Autodesk Inventor part; units mm, degrees
ref_plane "Work Plane1" through (0, 70, 0) normal (0, 1, 0) x (1, 0, 0)
ref_plane "YZ Plane" through (0, 0, 0) normal (1, 0, 0) x (0, 1, 0)
ref_plane "XZ Plane" through (0, 0, 0) normal (0, 1, 0) x (-1, 0, 0)
sketch "Sketch1" plane through (0, 0, 0) normal (0, 1, 0) x (-1, 0, 0)
  arc A0 (0, 30.16) -> (-3.6283, 29.941) centre (0, 0) ccw construction
  arc A1 (-26.9832, 26.9832) -> (-36.0277, -12.5774) centre (0, 0) ccw construction
  line L0 (38.16, 38.16) -> (0, 38.16) construction
  line L1 (-38.16, 38.16) -> (-38.16, -38.16)
  line L2 (-38.16, -38.16) -> (-4.1245, -38.16)
  line L3 (38.16, -38.16) -> (38.16, 38.16) construction
  line L4 (38.16, 38.16) -> (-21.3263, -21.3263) construction
  line L5 (-38.16, 38.16) -> (-21.3263, 21.3263) construction
  line L6 (0, 38.16) -> (-4.1245, 38.16) construction
  line L7 (0, -38.16) -> (38.16, -38.16) construction
  arc A2 (0, 38.16) -> (-26.9832, 26.9832) centre (0, 0) ccw construction
  arc A3 (-36.9415, -9.566) -> (-26.9832, -26.9832) centre (0, 0) ccw construction
  arc A4 (-26.9832, -26.9832) -> (0, -38.16) centre (0, 0) ccw construction
  arc A5 (0, -38.16) -> (0, 38.16) centre (0, 0) ccw construction
  line L8 (-21.3263, 21.3263) -> (38.16, -38.16) construction
  line L9 (-21.3263, -21.3263) -> (-38.16, -38.16) construction
  line L10 (0, 38.16) -> (0, 30.16) construction
  line L11 (0, -30.16) -> (0, -38.16) construction
  arc A6 (21.3263, 21.3263) -> (0, 30.16) centre (0, 0) ccw construction
  arc A7 (0, -30.16) -> (21.3263, 21.3263) centre (0, 0) ccw construction
  arc A8 (-6.0651, -37.6749) -> (-3.6283, -29.941) centre (-4.1245, -34.0355) ccw
  arc A9 (-3.6283, 29.941) -> (-6.0651, 37.6749) centre (-4.1245, 34.0355) ccw
  line L12 (-4.1245, -38.16) -> (0, -38.16) construction
  arc A10 (-3.6283, -29.941) -> (0, -30.16) centre (0, 0) ccw construction
  arc A11 (-3.6283, 29.941) -> (-3.6283, -29.941) centre (0, 0) ccw
  line L13 (-4.1245, 38.16) -> (-38.16, 38.16)
  arc A12 (-3.6283, -29.941) -> (-6.0651, -37.6749) centre (-4.1245, -34.0355) ccw construction
  arc A13 (-6.0651, 37.6749) -> (-3.6283, 29.941) centre (-4.1245, 34.0355) ccw construction
  dimension "d0" = 60.32
  dimension "d1" = 8
extrude "Extrusion1" add sketch "Sketch1" along normal blind 140
sketch "Sketch2" plane through (38.16, 0, 38.16) normal (1, 0, 0) x (0, 0, -1)
  line L0 (8.219, 140) -> (0, 140)
  line L1 (0, 140) -> (76.32, 0) construction
  line L2 (76.32, 140) -> (0, 0) construction
  circle A0 centre (38.16, 70) radius 25.4
  dimension "d15" = 50.8
extrude "Extrusion2" cut sketch "Sketch2" against normal up to next
ref_plane "Work Plane1" through (0, 70, 0) normal (0, 1, 0) x (1, 0, 0)
sketch "Sketch3" plane through (0, 70, 0) normal (0, 1, 0) x (1, 0, 0)
  line L0 (38.16, 38.16) -> (4.1245, 38.16)
  line L1 (38.16, 25.4) -> (16.2624, 25.4)
  line L2 (38.16, -38.16) -> (38.16, 38.16)
  line L3 (38.16, -25.4) -> (16.2624, -25.4)
  line L4 (4.1245, -38.16) -> (38.16, -38.16)
  line L5 (16.2624, 25.4) -> (38.16, 38.16) construction
  line L6 (38.16, 25.4) -> (16.2624, 38.16) construction
  line L7 (16.2624, -25.4) -> (38.16, -38.16) construction
  line L8 (38.16, -25.4) -> (16.2624, -38.16) construction
  circle A0 centre (27.2112, 31.78) radius 2.5
  circle A1 centre (27.2112, -31.78) radius 2.5
  dimension "d16" = 5
  dimension "d17" = 5
extrude "Extrusion3" cut sketch "Sketch3" along normal through all both and the other way through all
sketch "Sketch5" plane through (38.16, 0, 38.16) normal (1, 0, 0) x (0, 0, -1)
  circle A0 centre (38.16, 70) radius 25.4
  line L0 (0, 140) -> (76.32, 140)
  line L1 (0, 0) -> (76.32, 0)
  line L2 (38.16, 95.4) -> (38.16, 140) construction
  line L3 (38.16, 44.6) -> (38.16, 0) construction
  circle A1 centre (38.16, 112.125) radius 2.55
  circle A2 centre (38.16, 27.875) radius 2.55
  line L4 (38.16, 22.3) -> (38.16, 44.6) construction
  line L5 (38.16, 117.7) -> (38.16, 95.4) construction
  line L6 (38.16, 22.3) -> (38.16, 33.45)
  line L7 (38.16, 117.7) -> (38.16, 106.55)
  dimension "d18" = 5.1
  dimension "d19" = 5.1
extrude "Extrusion4" cut sketch "Sketch5" against normal up to next contours A1 L7 | L7 A1 | A2 L6 | L6 A2
ref_plane "Work Plane2" through (4.1245, 0, 0) normal (0, 0, 1) x (1, 0, 0)
sketch "Sketch7" plane through (38.16, 0, 38.16) normal (1, 0, 0) x (0, 0, -1)
  line L0 (0, 0) -> (0, 140) construction
  line L1 (0, 140) -> (0, 0) construction
  line L2 (0, 89) -> (0, 51)
  circle A0 centre (-4, 93) radius 4 construction
  circle A1 centre (-4, 93) radius 2.75
  circle A2 centre (-4, 85) radius 4 construction
  circle A3 centre (-4, 85) radius 2.75
  arc A4 (-12.9282, 85.5359) -> (-12.9282, 92.4641) centre (-10.9282, 89) ccw construction
  circle A5 centre (-10.9282, 89) radius 2.75
  line L3 (0, 70) -> (-10, 70) construction
  line L4 (0, 89) -> (-10, 89) construction
  line L5 (0, 78.0718) -> (-12.9282, 85.5359)
  line L6 (-12.9282, 92.4641) -> (0, 99.9282)
  arc A6 (-12.9282, 92.4641) -> (-12.9282, 85.5359) centre (-10.9282, 89) ccw
  circle A7 centre (-4, 47) radius 4 construction
  circle A8 centre (-4, 47) radius 2.75
  circle A9 centre (-4, 55) radius 4 construction
  circle A10 centre (-4, 55) radius 2.75
  arc A11 (-12.9282, 47.5359) -> (-12.9282, 54.4641) centre (-10.9282, 51) ccw construction
  circle A12 centre (-10.9282, 51) radius 2.75
  line L7 (0, 51) -> (-10, 51) construction
  line L8 (0, 61.9282) -> (-12.9282, 54.4641)
  line L9 (-12.9282, 47.5359) -> (0, 40.0718)
  arc A13 (-12.9282, 54.4641) -> (-12.9282, 47.5359) centre (-10.9282, 51) ccw
  line L10 (0, 89) -> (0, 99.9282)
  line L11 (0, 51) -> (0, 40.0718)
  point P0 (38.16, 0)
  dimension "d26" = 38
  dimension "d27" = 8
  dimension "d28" = 5.5
  dimension "d29" = 8
  dimension "d30" = 5.5
  dimension "d31" = 8
  dimension "d32" = 5.5
  dimension "d33" = 10
  dimension "d34" = 10
extrude "Extrusion6" add sketch "Sketch7" against normal blind 125.446
properties part number "Tubo Exterior" material "ABS Plastic"
Read the model definition and answer for the solid it produces. Units are mm, in the model's axes. A direction names the side the tool comes from. Coordinates: 2 decimals unless noted, no trailing zeros. Order: outer loops, then holes, each group sorted by start corner. A loop starts at its lowest first (then second) coordinate and runs counter-clockwise, first axis right, second up. Notation, with made-up numbers: (-1, -24) - (37, -24) arc R12 cw to (37, -6) - close; hole circle Ø7 at (67.5, 80). An arc over 180 degrees is marked (long way). Answer as a JSON object with one key per item and string values. Group by question number.
Item 1: Section C-C (y = 116.5) is taken. Give the vertices of the cut face in (x, z), plus the area to 3 significant figures.
Item 2: A tool of negligible diameter and unlimited length cuts with its end or side. For faces 1 (the face through (21, 70, 38.16)), 2 (the face through (-23.685, 57.727, 42.518)), from which of +Z, -Z, +X, -X, +Y, -Y can it reach the whole face along a straight path? Write none if from no direction.
Item 3: The mould has two halves that part along Z. Classify faces 3 (the face through (16.621, 53.464, -25.167)), 4 (the face through (32, 0, 1)), 5 (the face through (-23.68, 81.75, 44.53)): +Z half, -Z half, draft (parallel to the pull), parting line (faces both ways), or undercut.
Item 4: Flat-ended cylindrical pins translate along their axes: P1, Ø6, axis at x = -33.5, y = 45, coming from the -Z side; P2, Ø10, axis at x = 29, y = 122.5, coming from the +Z side; P3, Ø9, axis at y = 93, z = 42.16, coming from the +X side; P4, Ø3, axis at y = 17.5, z = 35.5, coming from the -X side. Find the tip coordinate at first contact, or state that the pin passes through.
Item 5: Consider probe 1 along Y at (x, z) = (36, 0) (3 decimals); probe 2 along Z at (x, y) = (13, 83); probe 3 along Z at (x, y) = (-4, 86.5). Determine where each line is inside the solid, lowest interval first. Write a range as from..to.
Item 6: Section B-B (z = 31.78) is taken. Give the vertices of the cut face in (x, y).
Item 7: Section A-A (x = -59) is taken. Give the vertices of the cut face in (y, z).
Item 8: Section D-D (z = 42.16) is taken. Give the vertices of the cut face in (x, y).
Results are:
{
 "1": {"outline": "(3.63, -29.94) arc R4.12 ccw to (4.12, -38.16) - (38.16, -38.16) - (38.16, 38.16) - (4.12, 38.16) arc R4.12 ccw to (3.63, 29.94) arc R30.16 cw to start; hole circle Ø5 at (27.21, -31.78); hole circle Ø5 at (27.21, 31.78)", "area": "1,430 mm^2"},
 "2": {"face 1": "+Z, +X, -X", "face 2": "+X, -X"},
 "3": {"face 3": "undercut", "face 4": "draft", "face 5": "+Z half"},
 "4": {"P1": "stops at z = 38.16", "P2": "stops at z = 38.16", "P3": "stops at x = 38.16", "P4": "stops at x = 0"},
 "5": {"probe 1": "y = 0..25.325, 30.425..44.6, 95.4..109.575, 114.675..140", "probe 2": "z = -38.16..-27.21, 27.21..40.27, 44.05..46.7", "probe 3": "z = 38.16..39.86, 44.46..47.94, 50.23..52.21"},
 "6": {"outline": "(0.67, 0) - (24.71, 0) - (24.71, 140) - (0.67, 140) - close; (29.71, 0) - (38.16, 0) - (38.16, 140) - (29.71, 140) - close"},
 "7": {"outline": "(40.07, 38.16) - (61.93, 38.16) - (54.46, 51.09) arc R4 ccw to (47.54, 51.09) - close; (78.07, 38.16) - (99.93, 38.16) - (92.46, 51.09) arc R4 ccw to (85.54, 51.09) - close; hole circle Ø5.5 at (47, 42.16); hole circle Ø5.5 at (51, 49.09); hole circle Ø5.5 at (55, 42.16); hole circle Ø5.5 at (85, 42.16); hole circle Ø5.5 at (89, 49.09); hole circle Ø5.5 at (93, 42.16)"},
 "8": {"outline": "(-87.29, 42.38) - (38.16, 42.38) - (38.16, 44.25) - (-87.29, 44.25) - close; (-87.29, 49.75) - (38.16, 49.75) - (38.16, 52.25) - (-87.29, 52.25) - close; (-87.29, 57.75) - (38.16, 57.75) - (38.16, 59.62) - (-87.29, 59.62) - close; (-87.29, 80.38) - (38.16, 80.38) - (38.16, 82.25) - (-87.29, 82.25) - close; (-87.29, 87.75) - (38.16, 87.75) - (38.16, 90.25) - (-87.29, 90.25) - close; (-87.29, 95.75) - (38.16, 95.75) - (38.16, 97.62) - (-87.29, 97.62) - close"}
}
